Source: CAD feature listing. Evaluate the final solid. Frame: model axes, mm. Give positions to 0.01 mm unless a question says otherwise; leave off trailing zeros. Write each loop counter-clockwise with the first axis right and the second up, starting at its lowest first coordinate (ties: lowest second). Pieces come first, ordered by that corner, then holes. Notation, with made-up numbers: (21.25, 41.5) -> (73.25, 41.5) arc R18 ccw to (73.25, 61.5) -> close; hole circle Ø3 at (-23.5, -28.75). An arc over 180 degrees is marked (long way). Answer as a JSON object with one key per item and string values. Group by question number.
Item 1: Section query A-A on y = -11. Return the cut outline in (x, z).
Item 2: Section query C-C on z = -2.5. Return the cut outline in (x, y), plus the area to 3 significant figures.
Item 3: Section query B-B on x = -31. Return the cut outline in (y, z).
Item 4: First-contact query: pin 1 Ø1 at (y, z) = (4, 7) entering from +X; pin 2 Ø1.5 at (y, z) = (-13.5, -4) entering from -X; pin 3 Ø4 at (x, z) = (1.5, -3) entering from +Y. Flat tips, straight axial feed; report the tip coordinate or a pass-through.
Item 5: Section query D-D on z = 6. Return the cut outline in (x, y).
Item 6: Ray query, probe 1 along Z at (x, y) = (-23, -13.5); probe 2 along X at (y, z) = (4.5, 9.75); probe 3 along Y at (x, z) = (-7, -0.5). Return the intervals inside material, ascending. Write a range as from..to.
from build123d import *

# Parameters (mm, degrees)
F1_DEPTH = 12.7
F2_W     = 25.4
F2_H     = 38.1
F3_DEPTH = 5.08


with BuildPart() as f1:
    # F0 (on Top) → F1 (new body)
    with BuildSketch(Plane.XY):
        Polygon((0, 76.2), (-38.1, -38.1), (38.1, -38.1), align=None)
    extrude(amount=F1_DEPTH)

    # F2 (on face) → F3 (join)
    with BuildSketch(Plane(origin=(0, 0, 0), x_dir=(1, 0, 0), z_dir=(0, 0, -1))):
        with Locations((0, 19.05)):
            Rectangle(F2_W, F2_H)
    extrude(amount=F3_DEPTH)


solid = f1.part
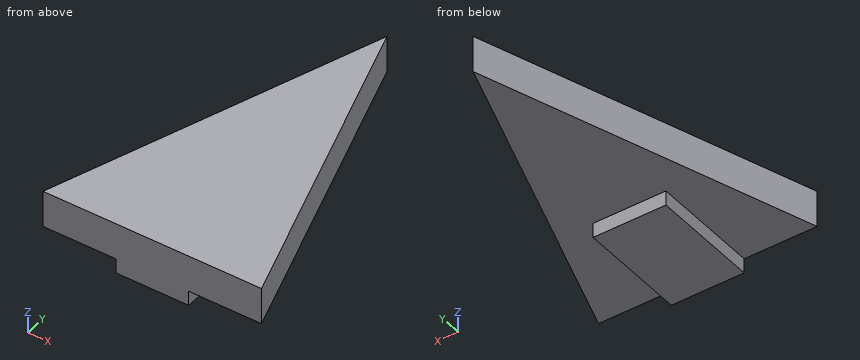
Worked answers:
{
 "1": {"outline": "(-29.07, 0) -> (-12.7, 0) -> (-12.7, -5.08) -> (12.7, -5.08) -> (12.7, 0) -> (29.07, 0) -> (29.07, 12.7) -> (-29.07, 12.7) -> close"},
 "2": {"outline": "(-12.7, -38.1) -> (12.7, -38.1) -> (12.7, 0) -> (-12.7, 0) -> close", "area": "968 mm^2"},
 "3": {"outline": "(-38.1, 0) -> (-16.8, 0) -> (-16.8, 12.7) -> (-38.1, 12.7) -> close"},
 "4": {"pin 1": "x = 24.23", "pin 2": "x = -12.7", "pin 3": "y = 0"},
 "5": {"outline": "(-38.1, -38.1) -> (38.1, -38.1) -> (0, 76.2) -> close"},
 "6": {"probe 1": "0..12.7", "probe 2": "-23.9..23.9", "probe 3": "-38.1..0"}
}
